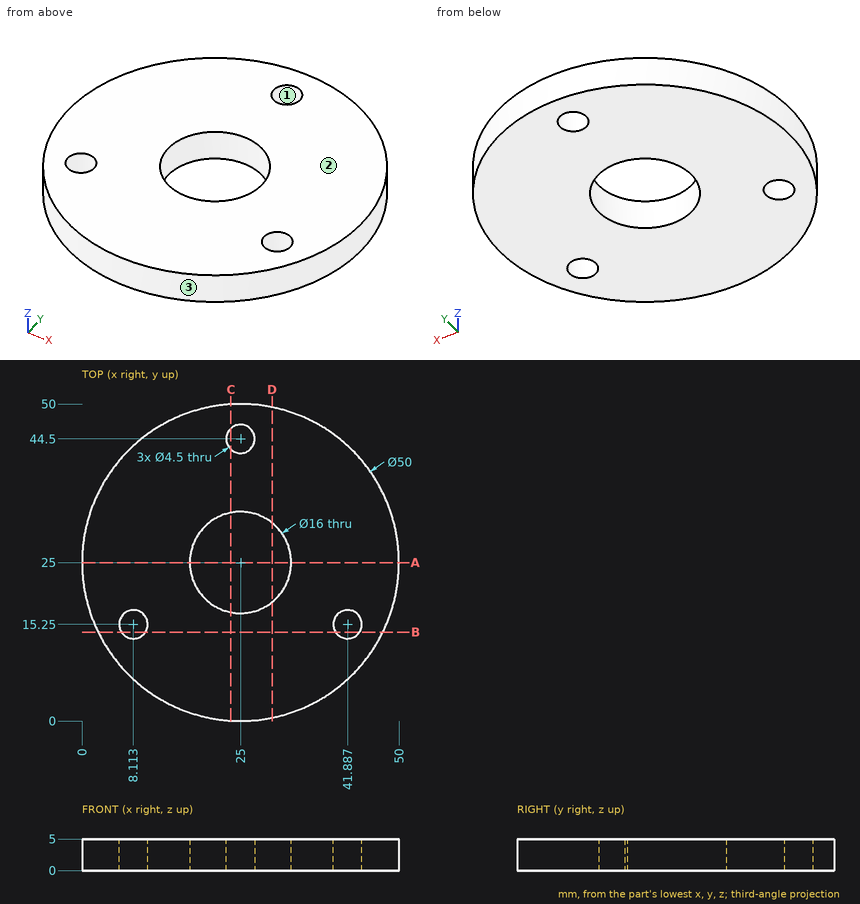
Geometry check sheet. Reference: drawing and pictorial views, mm from the part's lowest x, y, z. Give positions to 0.01 mm unless a question says otherwise; leave off trailing zeros. Order: outer loops, then holes, each group sorted by start corner. A loop starts at its lowest first (then second) coordinate and runs counter-clockwise, first axis right, second up.
1. Section check D-D, the plane x = 30. Enter the section's corners in (y, z) (1 decimal).
2. Gauge pin test, flat ends, axial feed: pin 1 Ø13 at (x, y) = (25, 25) entering from -Z; pin 2 Ø1.5 at (x, z) = (30, 4) entering from +Y; pin 3 Ø3 at (y, z) = (42.5, 2) entering from -X; pin 4 Ø1.5 at (x, z) = (6.5, 1) entering from +Y (1 decimal). Record the tip position at first contact, or that the pin passes through.
3. Section check C-C, the plane x = 23.5. Enter the section's corners in (y, z) (1 decimal), and give its area (3 significant figures).
4. Thickness scan on L1, parallel to Y at x = 25, z = 3.55; L2, parallel to Y at x = 26.5, z = 1.85 (1 decimal); L3, parallel to X at y = 21, z = 0.95. Record the ranges inside material, lowest first.
5. Section check A-A, the plane y = 25. Enter the section's corners in (x, z).
6. Section check B-B, the plane y = 14. Enter the section's corners in (x, z), and give its area (3 significant figures).
7. Release check for a two-part mould opening along Y. For the marked faces 1, 2 and 3 record: pulls with the +Y half, pulls with the -Y half, needs draft (parallel to the pull), parting line crosses it, or undercut.
Values follow:
1. outline: (0.5, 0) - (18.8, 0) - (18.8, 5) - (0.5, 5) - close; (31.2, 0) - (49.5, 0) - (49.5, 5) - (31.2, 5) - close
2. pin 1: passes through
2. pin 2: stops at y = 49.64
2. pin 3: stops at x = 5.79
2. pin 4: stops at y = 42.6
3. outline: (0, 0) - (17.1, 0) - (17.1, 5) - (0, 5) - close; (32.9, 0) - (42.8, 0) - (42.8, 5) - (32.9, 5) - close; (46.2, 0) - (50, 0) - (50, 5) - (46.2, 5) - close
3. area: 154 mm2
4. L1: y = 0 to 17, 33 to 42.25, 46.75 to 50
4. L2: y = 0 to 17.1, 32.9 to 42.8, 46.2 to 50
4. L3: x = 0.32 to 18.07, 31.93 to 49.68
5. outline: (0, 0) - (17, 0) - (17, 5) - (0, 5) - close; (33, 0) - (50, 0) - (50, 5) - (33, 5) - close
6. outline: (2.55, 0) - (6.24, 0) - (6.24, 5) - (2.55, 5) - close; (9.98, 0) - (40.02, 0) - (40.02, 5) - (9.98, 5) - close; (43.76, 0) - (47.45, 0) - (47.45, 5) - (43.76, 5) - close
6. area: 187 mm2
7. face 1: undercut
7. face 2: needs draft
7. face 3: parting line crosses it
